Here's how the part is built. I have some questions about the finished solid (model axes, mm). Give positions to 0.01 mm unless a question says otherwise; leave off trailing zeros. Write each loop counter-clockwise with the first axis right and the second up, starting at its lowest first coordinate (ties: lowest second). Pieces come first, ordered by that corner, then holes. Notation, with made-up numbers: (47.25, -4) - (62.25, -4) arc R32 cw to (62.25, 29) - close; hole circle Ø6 at (-20, 74). An arc over 180 degrees is marked (long way). Use a Markdown table: item, result.
```python
from build123d import *

# Parameters (mm, degrees)
EXTRUDE_1_DEPTH               = 8.2
SKETCH_2_OUTSIDE_W            = 31.148
SKETCH_2_OUTSIDE_H            = 28.828
SKETCH_2_OUTSIDE_R            = 7.5
CUT_EXTRUDE_1_DEPTH           = 8.2
CUT_EXTRUDE_1_DRAFT           = -23
SKETCH_3_OUTSIDE_W            = 31.148
SKETCH_3_OUTSIDE_H            = 28.828
SKETCH_3_OUTSIDE_R            = 7.5
CUT_EXTRUDE_2_DEPTH           = 8.2
CUT_EXTRUDE_2_DRAFT           = -23
HOLE_WIZARD_M10_1_D           = 8.5
HOLE_WIZARD_M10_1_CSINK_D     = 10.05
HOLE_WIZARD_M10_1_CSINK_ANGLE = 90


with BuildPart() as part:
    # 草图1 → 凸台-拉伸1 (new body)
    with BuildSketch(Plane(origin=(0, 0, 0), x_dir=(1, 0, 0), z_dir=(0, 1, 0))):
        Polygon((4.330127019, 7.5), (-4.330127019, 7.5), (-8.660254038, 0), (-4.330127019, -7.5), (4.330127019, -7.5), (8.660254038, 0), align=None)
    extrude(amount=EXTRUDE_1_DEPTH)


with BuildPart() as cut_extrude_1_tool:
    # 草图2 outside → 切除-拉伸1 (with draft: the straight prism first)
    with BuildSketch(Plane(origin=(0, 8.2, 0), x_dir=(1, 0, 0), z_dir=(0, 1, 0))):
        Rectangle(SKETCH_2_OUTSIDE_W, SKETCH_2_OUTSIDE_H)
        Circle(SKETCH_2_OUTSIDE_R, mode=Mode.SUBTRACT)
    extrude(amount=-CUT_EXTRUDE_1_DEPTH)
    # 切除-拉伸1: the draft: its side faces are tilted about the plane it starts from
    cut_extrude_1_sides = [cut_extrude_1_tool.faces().sort_by_distance(p)[0] for p in [
        (0, 4.1, 14.414),
        (15.574, 4.1, 0),
        (0, 4.1, -14.414),
        (-15.574, 4.1, 0),
        (-7.5, 4.1, 0),
    ]]
    draft(cut_extrude_1_sides, Plane(origin=(0, 8.2, 0), x_dir=(1, 0, 0), z_dir=(0, 1, 0)), CUT_EXTRUDE_1_DRAFT)


with BuildPart() as part_1:
    add(part.part)

    # 切除-拉伸1: cut by cut_extrude_1_tool
    add(cut_extrude_1_tool.part, mode=Mode.SUBTRACT)


with BuildPart() as cut_extrude_2_tool:
    # 草图3 outside → 切除-拉伸2 (with draft: the straight prism first)
    with BuildSketch(Plane.XZ):
        Rectangle(SKETCH_3_OUTSIDE_W, SKETCH_3_OUTSIDE_H)
        Circle(SKETCH_3_OUTSIDE_R, mode=Mode.SUBTRACT)
    extrude(amount=-CUT_EXTRUDE_2_DEPTH)
    # 切除-拉伸2: the draft: its side faces are tilted about the plane it starts from
    cut_extrude_2_sides = [cut_extrude_2_tool.faces().sort_by_distance(p)[0] for p in [
        (0, 4.1, -14.414),
        (15.574, 4.1, 0),
        (0, 4.1, 14.414),
        (-15.574, 4.1, 0),
        (-7.5, 4.1, 0),
    ]]
    draft(cut_extrude_2_sides, Plane.XZ, CUT_EXTRUDE_2_DRAFT)


with BuildPart() as part_2:
    add(part_1.part)

    # 切除-拉伸2: cut by cut_extrude_2_tool
    add(cut_extrude_2_tool.part, mode=Mode.SUBTRACT)

    # M10 螺纹孔1 (through all)
    with Locations(Plane(origin=(0, 8.2, 0), x_dir=(1, 0, 0), z_dir=(0, 1, 0))):
        with Locations((0, 0)):
            CounterSinkHole(HOLE_WIZARD_M10_1_D / 2, HOLE_WIZARD_M10_1_CSINK_D / 2, counter_sink_angle=HOLE_WIZARD_M10_1_CSINK_ANGLE)


solid = part_2.part
```
Item 1: If we section it at B-B, the plane y = 5.75: Write out the boundary of the cut face in (x, z), plus the area to 3 significant figures.
Values:
| item | result |
|---|---|
| outline | (-8.54, -0.21) - (-4.45, -7.29) arc R8.54 ccw to (-4.08, -7.5) - (4.08, -7.5) arc R8.54 ccw to (4.45, -7.29) - (8.54, -0.21) arc R8.54 ccw to (8.54, 0.21) - (4.45, 7.29) arc R8.54 ccw to (4.08, 7.5) - (-4.08, 7.5) arc R8.54 ccw to (-4.45, 7.29) - (-8.54, 0.21) arc R8.54 ccw to start; hole circle Ø8.5 at (0, 0) |
| area | 138 mm2 |
Item 2: Will these pins go through, and if not, where does the flat tip stop? pin 1 Ø5 at (x, z) = (-0.5, 2.5) entering from -Y; pin 2 Ø4 at (x, y) = (6.5, 6) entering from +Z.
Values:
| item | result |
|---|---|
| pin 1 | stops at y = 0 |
| pin 2 | stops at z = 7.2 |
Item 3: I need wall thicknesses on line 1 along Z through (x, y) = (0, 5.5); line 2 along X through (y, z) = (3.75, 3.75); line 3 along Z through (x, y) = (-3.25, 4.75). Which ranges of each line are inside material? Lowest first, please. Write a range as [from, to].
Values:
| item | result |
|---|---|
| line 1 | z = [-7.5, -4.25], [4.25, 7.5] |
| line 2 | x = [-6.5, -2], [2, 6.5] |
| line 3 | z = [-7.5, -2.74], [2.74, 7.5] |
Item 4: If we section it at A-A, the plane y = 3.75: Write out the boundary of the cut face in (x, z), plus the area to 3 significant figures.
Values:
| item | result |
|---|---|
| outline | (-8.66, 0) - (-4.33, -7.5) - (4.33, -7.5) - (8.66, 0) - (4.33, 7.5) - (-4.33, 7.5) - close; hole circle Ø8.5 at (0, 0) |
| area | 138 mm2 |
